```python
from build123d import *

# Parameters (mm, degrees)
F0_R         = 1.5875
F1_DEPTH     = 304.8
F3_DEPTH     = 1.0795
F4_T4_DEPTH  = 15.027948453
F4_S5_R      = 1.5875
F4_T6_DEPTH  = 9
F4_T10_DEPTH = 15.027948453
F4_S11_R     = 1.5875
F4_T12_DEPTH = 9
F5_R         = 1.5875
F6_DEPTH     = 2.6680001


# Not quite as in the source:
# - a fillet or chamfer that OpenCascade refuses, or shapes differently, is made with other operations: its cross-section is extruded or revolved along the edge and cut away or added


with BuildPart() as f1:
    # F0 (on Right) → F1 (new body, symmetric)
    with BuildSketch(Plane.YZ):
        Circle(F0_R)
    extrude(amount=F1_DEPTH, both=True)

    # F2 (on Front) → F3 (join, symmetric)
    with BuildSketch(Plane.XZ):
        with BuildLine():
            Line((304.7385620117, -2.3473887456), (317.4385620117, -2.3473887456))
            ThreePointArc((317.4385620117, -2.3473887456), (318.7856004299, -1.7894271638), (319.3435620117, -0.4423887456))
            Line((319.3435620117, -0.4423887456), (319.3435620117, 0.4423887456))
            ThreePointArc((319.3435620117, 0.4423887456), (318.7856004299, 1.7894271638), (317.4385620117, 2.3473887456))
            Line((317.4385620117, 2.3473887456), (304.7385620117, 2.3473887456))
            ThreePointArc((304.7385620117, 2.3473887456), (303.3915235936, 1.7894271638), (302.8335620117, 0.4423887456))
            Line((302.8335620117, 0.4423887456), (302.8335620117, -0.4423887456))
            ThreePointArc((302.8335620117, -0.4423887456), (303.3915235936, -1.7894271638), (304.7385620117, -2.3473887456))
        make_face()
    extrude(amount=F3_DEPTH, both=True)

    # F4: fillet of radius 2.54 on 2 edges, made by hand


with BuildPart() as f4_tool2:
    # F4_s3 → F4_t4 (new body)
    with BuildSketch(Plane.XY.offset(7.5139742265)):
        with BuildLine():
            ThreePointArc((307.34, -1.0795), (305.5439487758, -1.8234487758), (304.8, -3.6195))
            Line((304.8, -3.6195), (304.8, -1.0795))
            Line((304.8, -1.0795), (307.34, -1.0795))
        make_face()
    extrude(amount=-F4_T4_DEPTH)

    # F4_s5 → F4_t6 (intersect, symmetric)
    with BuildSketch(Plane.YZ.offset(306.1)):
        Circle(F4_S5_R)
    extrude(amount=F4_T6_DEPTH, both=True, mode=Mode.INTERSECT)


with BuildPart() as f1_1:
    add(f1.part)

    # F4_t1: union F4_tool2
    add(f4_tool2.part)


with BuildPart() as f4_tool8:
    # F4_s9 → F4_t10 (new body)
    with BuildSketch(Plane.XY.offset(7.5139742265)):
        with BuildLine():
            ThreePointArc((304.8, 3.6195), (305.5439487758, 1.8234487758), (307.34, 1.0795))
            Line((307.34, 1.0795), (304.8, 1.0795))
            Line((304.8, 1.0795), (304.8, 3.6195))
        make_face()
    extrude(amount=-F4_T10_DEPTH)

    # F4_s11 → F4_t12 (intersect, symmetric)
    with BuildSketch(Plane.YZ.offset(306.1)):
        Circle(F4_S11_R)
    extrude(amount=F4_T12_DEPTH, both=True, mode=Mode.INTERSECT)


with BuildPart() as f1_2:
    add(f1_1.part)

    # F4_t7: union F4_tool8
    add(f4_tool8.part)

    # F5 (on face) → F6 (cut, through all)
    with BuildSketch(Plane.XZ.offset(1.0795)):
        with Locations((316.8214559555, 0)):
            Circle(F5_R)
    extrude(amount=-F6_DEPTH, mode=Mode.SUBTRACT)


solid = f1_2.part
```
Source: CAD feature listing. Evaluate the final solid. Frame: model axes, mm. Give positions to 0.01 mm unless a question says otherwise; leave off trailing zeros. Write each loop counter-clockwise with the first axis right and the second up, starting at its lowest first coordinate (ties: lowest second). Pieces come first, ordered by that corner, then holes. Notation, with made-up numbers: (-34, 57) - (-26, 57) arc R19 cw to (-26, 70) - close; hole circle Ø11 at (-5.5, 38.5). An arc over 180 degrees is marked (long way). One line per item, written item: value. Start each with the question number.
Q1. First-contact query: pin 1 Ø1.5 at (x, y) = (253.5, -0.5) entering from +Z; pin 2 Ø1.4 at (x, z) = (313.5, 1) entering from -Y. Flat tips, straight axial feed; report the tip coordinate or a pass-through.
Q2. Material intervals for probe 1 along Y at (x, z) = (-159, 0.1); probe 2 along Y at (x, z) = (-150, -1.1); probe 3 along Z at (x, y) = (109, -0.25), sorted ascending. Write a range as from..to.
Q3. Section query B-B, the plane x = 168. Return the cut outline in (y, z) (1 decimal).
Q4. Section query A-A, the plane y = 0. Return the cut outline in (x, z) (1 decimal).
Answer:
1. pin 1: stops at z = 1.59
1. pin 2: stops at y = -1.08
2. probe 1: y = -1.58..1.58
2. probe 2: y = -1.14..1.14
2. probe 3: z = -1.57..1.57
3. outline: circle Ø3.2 at (0, 0)
4. outline: (-304.8, -1.6) - (303.2, -1.6) arc R1.9 ccw to (304.7, -2.3) - (317.4, -2.3) arc R1.9 ccw to (319.3, -0.4) - (319.3, 0.4) arc R1.9 ccw to (317.4, 2.3) - (304.7, 2.3) arc R1.9 ccw to (303.2, 1.6) - (-304.8, 1.6) - close; hole circle Ø3.2 at (316.8, 0)
